Input: part model. Units: mm. Frame: model coordinates. Face numbers are marked on the shaded views. A direction names the side the tool comes from. Round coordinates to 2 decimals unless told otherwise and drop trailing zeros. Loops run counter-clockwise (first coordinate to the right, second up) from the corner with the lowest first, then second, coordinate; pieces in that order, holes last. Notation, with made-up numbers: (76, -28.75) - (112, -28.75) arc R18 ccw to (112, -5.75) - close; hole circle Ø1 at (19, 61). An arc over 180 degrees is marked (long way). Use CSV: the item, a comma, the result in double quotes. Start each with the question number.
1. Material intervals for probe 1 along X at (y, z) = (-22, 18); probe 2 along X at (y, z) = (-64, 12.25), sorted ascending. Write a range as from..to.
2. Cut plane C-C (z = 19.5). Return loops of the section in (x, y).
3. Pin query (flat end, axial travel): P1, Ø7.5, axis at x = 29.5, z = 17, coming from the +Y side; P2, Ø7.5, axis at y = 12, z = 12, coming from the +X side; P3, Ø7.5, axis at x = 18.5, z = 15.5, coming from the -Y side. Return the tip coordinate at first contact, or that it passes through.
4. Access query for the marked faces 4, 5 and 6. Directions: +Z, -Z, +X, -X, +Y, -Y. A direction counts if a zero-diameter tool reaches every point of the face in a straight line with its end or side. Return the directions, or none.
5. Pull-direction query (X, two-part tool) for the marked faces 1, 2 and 3; classes: +X half, -X half, draft (parallel to the pull), parting line (faces both ways), or undercut.
6. Cut plane A-A (x = -11). Return loops of the section in (y, z).
```python
from build123d import *

# Parameters (mm, degrees)
F1_DEPTH = 25
F2_DEPTH = 0.6


with BuildPart() as f1:
    # F0 (on Top) → F1 (new body)
    with BuildSketch(Plane.XY):
        with BuildLine():
            Line((69.5, -62.5), (69.5, 62.5))
            ThreePointArc((69.5, 62.5), (67.449747, 67.449747), (62.5, 69.5))
            Line((62.5, 69.5), (-62.5, 69.5))
            ThreePointArc((-62.5, 69.5), (-67.449747, 67.449747), (-69.5, 62.5))
            Line((-69.5, 62.5), (-69.5, -62.5))
            ThreePointArc((-69.5, -62.5), (-67.449747, -67.449747), (-62.5, -69.5))
            Line((-62.5, -69.5), (62.5, -69.5))
            ThreePointArc((62.5, -69.5), (67.449747, -67.449747), (69.5, -62.5))
        make_face()
        with BuildLine():
            Line((-62.5, 67.5), (62.5, 67.5))
            ThreePointArc((62.5, 67.5), (66.035534, 66.035534), (67.5, 62.5))
            Line((67.5, 62.5), (67.5, -62.5))
            ThreePointArc((67.5, -62.5), (66.035534, -66.035534), (62.5, -67.5))
            Line((62.5, -67.5), (-62.5, -67.5))
            ThreePointArc((-62.5, -67.5), (-66.035534, -66.035534), (-67.5, -62.5))
            Line((-67.5, -62.5), (-67.5, 62.5))
            ThreePointArc((-67.5, 62.5), (-66.035534, 66.035534), (-62.5, 67.5))
        make_face(mode=Mode.SUBTRACT)
    extrude(amount=F1_DEPTH)

    # F0 (on Top) → F2 (join)
    with BuildSketch(Plane.XY):
        with BuildLine():
            Line((74.5, -62.5), (74.5, 62.5))
            ThreePointArc((74.5, 62.5), (70.985281, 70.985281), (62.5, 74.5))
            Line((62.5, 74.5), (-62.5, 74.5))
            ThreePointArc((-62.5, 74.5), (-70.985281, 70.985281), (-74.5, 62.5))
            Line((-74.5, 62.5), (-74.5, -62.5))
            ThreePointArc((-74.5, -62.5), (-70.985281, -70.985281), (-62.5, -74.5))
            Line((-62.5, -74.5), (62.5, -74.5))
            ThreePointArc((62.5, -74.5), (70.985281, -70.985281), (74.5, -62.5))
        make_face()
        with BuildLine():
            ThreePointArc((62.5, 69.5), (67.449747, 67.449747), (69.5, 62.5))
            Line((69.5, 62.5), (69.5, -62.5))
            ThreePointArc((69.5, -62.5), (67.449747, -67.449747), (62.5, -69.5))
            Line((62.5, -69.5), (-62.5, -69.5))
            ThreePointArc((-62.5, -69.5), (-67.449747, -67.449747), (-69.5, -62.5))
            Line((-69.5, -62.5), (-69.5, 62.5))
            ThreePointArc((-69.5, 62.5), (-67.449747, 67.449747), (-62.5, 69.5))
            Line((-62.5, 69.5), (62.5, 69.5))
        make_face(mode=Mode.SUBTRACT)
    extrude(amount=F2_DEPTH)


solid = f1.part
```
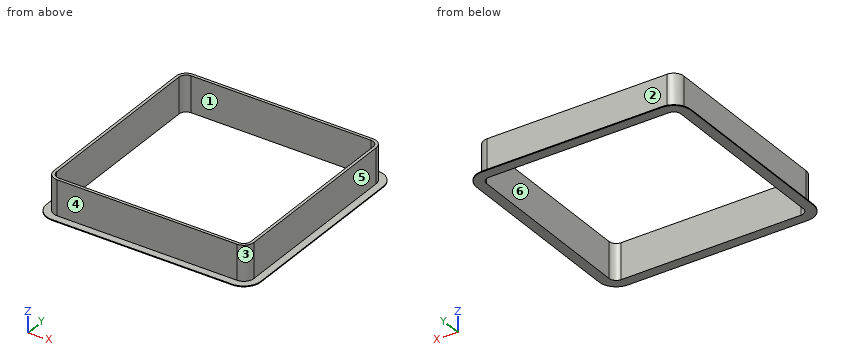
Established:
1,probe 1,"x = -69.5..-67.5, 67.5..69.5"
1,probe 2,"x = -69.34..-67.27, 67.27..69.34"
2,outline,"(-69.5, -62.5) arc R7 ccw to (-62.5, -69.5) - (62.5, -69.5) arc R7 ccw to (69.5, -62.5) - (69.5, 62.5) arc R7 ccw to (62.5, 69.5) - (-62.5, 69.5) arc R7 ccw to (-69.5, 62.5) - close; hole (-67.5, -62.5) arc R5 ccw to (-62.5, -67.5) - (62.5, -67.5) arc R5 ccw to (67.5, -62.5) - (67.5, 62.5) arc R5 ccw to (62.5, 67.5) - (-62.5, 67.5) arc R5 ccw to (-67.5, 62.5) - close"
3,P1,"stops at y = 69.5"
3,P2,"stops at x = 69.5"
3,P3,"stops at y = -69.5"
4,face 4,"+Z, +X, -X, -Y"
4,face 5,"+Z, +X, +Y, -Y"
4,face 6,"+Z, -Z"
5,face 1,"undercut"
5,face 2,"draft"
5,face 3,"+X half"
6,outline,"(-74.5, 0) - (-67.5, 0) - (-67.5, 25) - (-69.5, 25) - (-69.5, 0.6) - (-74.5, 0.6) - close; (67.5, 0) - (74.5, 0) - (74.5, 0.6) - (69.5, 0.6) - (69.5, 25) - (67.5, 25) - close"
